Autodesk Inventor part; units mm, degrees
ref_plane "YZ Plane" through (0, 0, 0) normal (1, 0, 0) x (0, 1, 0)
ref_plane "XZ Plane" through (0, 0, 0) normal (0, 1, 0) x (-1, 0, 0)
ref_plane "XY Plane" through (0, 0, 0) normal (0, 0, 1) x (1, 0, 0)
sketch "Sketch1" plane through (0, 0, 0) normal (0, 0, 1) x (1, 0, 0)
  circle A0 centre (0, 0) radius 3.4
  line L0 (0, 0) -> (20, 20) construction
  line L1 (0, 0) -> (28.2843, 0) construction
  line L2 (20, 20) -> (4.15, 20)
  line L3 (4.15, 20) -> (4.15, 15.5)
  line L4 (4.15, 15.5) -> (7.1, 15.5)
  line L5 (7.1, 15.5) -> (7.1, 18)
  line L6 (7.1, 18) -> (10.25, 18)
  line L7 (10.25, 18) -> (10.25, 14)
  line L8 (0, 0) -> (0, 26.1056) construction
  line L9 (10.25, 14) -> (2.3, 6.05)
  line L10 (2.3, 6.05) -> (0, 6.05)
  circle A1 centre (15, 15) radius 3
  line L11 (20, 20) -> (20, 4.15)
  line L12 (20, 4.15) -> (15.5, 4.15)
  line L13 (15.5, 4.15) -> (15.5, 7.1)
  line L14 (15.5, 7.1) -> (18, 7.1)
  line L15 (18, 7.1) -> (18, 10.25)
  line L16 (18, 10.25) -> (14, 10.25)
  line L17 (14, 10.25) -> (6.05, 2.3)
  line L18 (6.05, 2.3) -> (6.05, 0)
  line L19 (-2.3, 6.05) -> (0, 6.05)
  line L20 (-10.25, 14) -> (-2.3, 6.05)
  line L21 (-10.25, 18) -> (-10.25, 14)
  line L22 (-4.15, 15.5) -> (-7.1, 15.5)
  line L23 (-7.1, 15.5) -> (-7.1, 18)
  line L24 (-7.1, 18) -> (-10.25, 18)
  line L25 (-4.15, 20) -> (-4.15, 15.5)
  line L26 (-20, 20) -> (-4.15, 20)
  circle A2 centre (-15, 15) radius 3
  line L27 (-20, 20) -> (-20, 4.15)
  line L28 (-14, 10.25) -> (-6.05, 2.3)
  line L29 (-18, 7.1) -> (-18, 10.25)
  line L30 (-18, 10.25) -> (-14, 10.25)
  line L31 (-20, 4.15) -> (-15.5, 4.15)
  line L32 (-15.5, 4.15) -> (-15.5, 7.1)
  line L33 (-15.5, 7.1) -> (-18, 7.1)
  line L34 (-6.05, 2.3) -> (-6.05, 0)
  line L35 (-6.05, -2.3) -> (-6.05, 0)
  line L36 (-14, -10.25) -> (-6.05, -2.3)
  line L37 (-18, -10.25) -> (-14, -10.25)
  line L38 (-15.5, -4.15) -> (-15.5, -7.1)
  line L39 (-15.5, -7.1) -> (-18, -7.1)
  line L40 (-18, -7.1) -> (-18, -10.25)
  line L41 (-20, -4.15) -> (-15.5, -4.15)
  line L42 (-20, -20) -> (-20, -4.15)
  circle A3 centre (-15, -15) radius 3
  line L43 (-20, -20) -> (-4.15, -20)
  line L44 (-10.25, -14) -> (-2.3, -6.05)
  line L45 (-7.1, -18) -> (-10.25, -18)
  line L46 (-10.25, -18) -> (-10.25, -14)
  line L47 (-4.15, -20) -> (-4.15, -15.5)
  line L48 (-4.15, -15.5) -> (-7.1, -15.5)
  line L49 (-7.1, -15.5) -> (-7.1, -18)
  line L50 (-2.3, -6.05) -> (0, -6.05)
  line L51 (2.3, -6.05) -> (0, -6.05)
  line L52 (10.25, -14) -> (2.3, -6.05)
  line L53 (10.25, -18) -> (10.25, -14)
  line L54 (4.15, -15.5) -> (7.1, -15.5)
  line L55 (7.1, -15.5) -> (7.1, -18)
  line L56 (7.1, -18) -> (10.25, -18)
  line L57 (4.15, -20) -> (4.15, -15.5)
  line L58 (20, -20) -> (4.15, -20)
  circle A4 centre (15, -15) radius 3
  line L59 (20, -20) -> (20, -4.15)
  line L60 (14, -10.25) -> (6.05, -2.3)
  line L61 (18, -7.1) -> (18, -10.25)
  line L62 (18, -10.25) -> (14, -10.25)
  line L63 (20, -4.15) -> (15.5, -4.15)
  line L64 (15.5, -4.15) -> (15.5, -7.1)
  line L65 (15.5, -7.1) -> (18, -7.1)
  line L66 (6.05, -2.3) -> (6.05, 0)
  point P0 (0, 6.05)
  point P1 (-6.05, 0)
  point P2 (0, -6.05)
  dimension "d0" = 6.8
  dimension "d1" = 45
  dimension "d2" = 20
  dimension "d3" = 6
  dimension "d4" = 15
  dimension "d5" = 10.25
  dimension "d6" = 7.1
  dimension "d7" = 4.15
  dimension "d8" = 4.5
  dimension "d9" = 2
  dimension "d10" = 13.95
  dimension "d11" = 6
  dimension "d14" = 360
extrude "Extrusion1" add sketch "Sketch1" along normal blind 100.14
ref_plane "Work Plane1" through (0, 0, 50.07) normal (0, 0, 1) x (1, 0, 0)
sketch "Sketch2" plane through (20, -20, 0) normal (1, 0, 0) x (0, 0, -1)
  line L0 (-45.845, 6) -> (-45.845, 10.92)
  line L1 (-45.845, 10.92) -> (-54.295, 10.92)
  line L2 (-54.295, 10.92) -> (-54.295, 6)
  line L3 (-54.295, 6) -> (-45.845, 6)
  line L4 (-45.57, 11.195) -> (-45.57, 5.725)
  line L5 (-45.57, 5.725) -> (-54.57, 5.725)
  line L6 (-54.57, 5.725) -> (-54.57, 11.195)
  line L7 (-54.57, 11.195) -> (-45.57, 11.195)
  line L8 (0, 15.85) -> (-100.14, 15.85)
  line L9 (-54.57, 11.195) -> (-54.57, 15.85)
  line L10 (-45.57, 11.195) -> (-45.57, 15.85)
  point P0 (0, 20)
  dimension "d18" = 0.275
extrude "Extrusion2" cut sketch "Sketch2" against normal blind 6 contours L3 L2 L1 L0 | L4 L5 L6 L7 | L7 L9 L8 L10
properties part number "Aluminum_Profile_4040_100.14mm_top" material "Aluminum 6061-AHC"
Verification items for the finished model (mm, model axes). A direction names the side the tool comes from. Coordinates: 2 decimals unless noted, no trailing zeros. Order: outer loops, then holes, each group sorted by start corner. A loop starts at its lowest first (then second) coordinate and runs counter-clockwise, first axis right, second up. Notation, with made-up numbers: (33.25, 42.5) -> (54.25, 42.5) arc R23 cw to (54.25, 60.5) -> close; hole circle Ø7 at (38, 15). An arc over 180 degrees is marked (long way). Use CSV: the item, a comma, the result in double quotes. Start each with the question number.
Q1. Section check B-B, the plane z = 28. Give the number of separate pieces and of enclosed holes in the cut face, and give its area (3 significant figures).
Q2. Thickness scan on line 1 along Y through (x, z) = (-15, 34.5); line 2 along Y through (x, z) = (15, 46); line 3 along X through (y, z) = (13, 79). Record the ranges inside material, lowest first.
Q3. Section check A-A, the plane x = 0. Record the cut outline in (y, z), and give its area (3 significant figures).
Q4. Tool access check on faces 1 (the flat face through (17, -7.1, 77)), 2 (the flat face through (18, -4.15, 77)), 3 (the flat face through (-18, -4.15, 49)). Record the directions out of +Z, -Z, +X, -X, +Y, -Y that give a thin tool (end or side, any length) a straight path to the whole face; none if there is none.
Q5. Draft check along Y on faces 4 (the flat face through (-10.25, 16, 49)), 5 (the flat face through (12, -20, 49)). Enter one of: +Y half, -Y half, draft (parallel to the pull), parting line (faces both ways), or undercut.
Returned:
1,separate pieces,"1"
1,enclosed holes,"5"
1,area,"716 mm^2"
2,line 1,"y = -20 to -18, -12 to -10.25, 10.25 to 12, 18 to 20"
2,line 2,"y = -20 to -18, 10.25 to 12, 18 to 20"
2,line 3,"x = -20 to -17.24, -12.76 to -9.25, 9.25 to 12.76, 17.24 to 20"
3,outline,"(-6.05, 0) -> (-3.4, 0) -> (-3.4, 100.14) -> (-6.05, 100.14) -> close; (3.4, 0) -> (6.05, 0) -> (6.05, 100.14) -> (3.4, 100.14) -> close"
3,area,"531 mm^2"
4,face 1,"+Z, -Z"
4,face 2,"+Z, -Z, +X"
4,face 3,"+Z, -Z, -X"
5,face 4,"undercut"
5,face 5,"-Y half"
